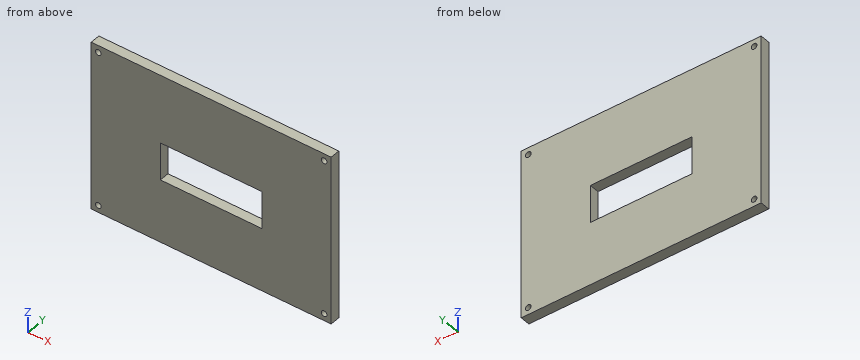
```python
from build123d import *

# Parameters (mm, degrees)
SKETCH1_W           = 170
SKETCH1_H           = 120
BOSS_EXTRUDE1_DEPTH = 7
SKETCH2_W           = 72
SKETCH2_H           = 26.620567464
CUT_EXTRUDE1_DEPTH  = 7
SKETCH3_R           = 2
CUT_EXTRUDE5_DEPTH  = 7
SKETCH7_R           = 2
CUT_EXTRUDE7_DEPTH  = 10
SKETCH6_R           = 2
CUT_EXTRUDE10_DEPTH = 10
SKETCH9_R           = 2
CUT_EXTRUDE11_DEPTH = 10


with BuildPart() as part:
    # Sketch1 → Boss-Extrude1 (new body)
    with BuildSketch(Plane(origin=(0, 0, 0), x_dir=(1, 0, 0), z_dir=(0, 1, 0))):
        Rectangle(SKETCH1_W, SKETCH1_H)
    extrude(amount=BOSS_EXTRUDE1_DEPTH)

    # Sketch2 → Cut-Extrude1 (cut)
    with BuildSketch(Plane(origin=(0, 7, 0), x_dir=(1, 0, 0), z_dir=(0, 1, 0))):
        with Locations((0, 1.926488435)):
            Rectangle(SKETCH2_W, SKETCH2_H)
    extrude(amount=-CUT_EXTRUDE1_DEPTH, mode=Mode.SUBTRACT)

    # Sketch3 → Cut-Extrude5 (cut)
    with BuildSketch(Plane(origin=(0, 7, 0), x_dir=(1, 0, 0), z_dir=(0, 1, 0))):
        with Locations((-80, 55)):
            Circle(SKETCH3_R)
    extrude(amount=-CUT_EXTRUDE5_DEPTH, mode=Mode.SUBTRACT)

    # Sketch7 → Cut-Extrude7 (cut)
    with BuildSketch(Plane(origin=(0, 7, 0), x_dir=(1, 0, 0), z_dir=(0, 1, 0))):
        with Locations((-80, -55)):
            Circle(SKETCH7_R)
    extrude(amount=-CUT_EXTRUDE7_DEPTH, mode=Mode.SUBTRACT)

    # Sketch6 → Cut-Extrude10 (cut)
    with BuildSketch(Plane(origin=(0, 7, 0), x_dir=(1, 0, 0), z_dir=(0, 1, 0))):
        with Locations((80, 55)):
            Circle(SKETCH6_R)
    extrude(amount=-CUT_EXTRUDE10_DEPTH, mode=Mode.SUBTRACT)

    # Sketch9 → Cut-Extrude11 (cut)
    with BuildSketch(Plane(origin=(0, 7, 0), x_dir=(1, 0, 0), z_dir=(0, 1, 0))):
        with Locations((80, -55)):
            Circle(SKETCH9_R)
    extrude(amount=-CUT_EXTRUDE11_DEPTH, mode=Mode.SUBTRACT)


solid = part.part
```
Could you check a few things on this model? Use its own coordinates, in mm. Round coordinates to 2 decimals unless told otherwise and drop trailing zeros. Order: outer loops, then holes, each group sorted by start corner. A loop starts at its lowest first (then second) coordinate and runs counter-clockwise, first axis right, second up. Notation, with made-up numbers: M -17,69 L 21,69 A26 ccw 21,83 Z; hole C 10.25,75 d4. An arc over 180 degrees is marked long. One line per question, with ' | ' between items. Start each with the question number.
(1) Suppose I cut it at C-C on y = 2.25. List the corners of the cut face in (x, z) for me, then the cut area to 3 significant figures.
(2) Suppose I cut it at A-A on z = -1. List the corners of the cut face in (x, y) for me.
(3) Suppose I cut it at B-B on x = 13. List the corners of the cut face in (y, z) for me, then the cut area to 3 significant figures.
(4) Please list where these lines run through material, in increasing order: line 1 along Z through (x, y) = (-80, 2.5); line 2 along X through (y, z) = (1.5, -55); line 3 along Z through (x, y) = (13, 3.5).
(5) For P1, Ø3, axis at x = -80, z = 55, coming from the +Y side, with a flat end and sliding along its axis, tell me the tip position at first contact or that it passes through.
(6) Suppose I cut it at D-D on x = -80. List the corners of the cut face in (y, z) for me.
Geometry results:
1) outline: M -85,-60 L 85,-60 L 85,60 L -85,60 Z; hole C -80,-55 d4; hole C -80,55 d4; hole M -36,-15.24 L 36,-15.24 L 36,11.38 L -36,11.38 Z; hole C 80,-55 d4; hole C 80,55 d4 | area: 18,400 mm²
2) outline: M -85,0 L -36,0 L -36,7 L -85,7 Z; M 36,0 L 85,0 L 85,7 L 36,7 Z
3) outline: M 0,-60 L 7,-60 L 7,-15.24 L 0,-15.24 Z; M 0,11.38 L 7,11.38 L 7,60 L 0,60 Z | area: 654 mm²
4) line 1: -60 to -57, -53 to 53, 57 to 60 | line 2: -85 to -82, -78 to 78, 82 to 85 | line 3: -60 to -15.24, 11.38 to 60
5) P1: through
6) outline: M 0,-60 L 7,-60 L 7,-57 L 0,-57 Z; M 0,-53 L 7,-53 L 7,53 L 0,53 Z; M 0,57 L 7,57 L 7,60 L 0,60 Z
